```python
from build123d import *

# Parameters (mm, degrees)
F1_DEPTH = 35
F3_DEPTH = 70
F4_R     = 15
F5_DEPTH = 80.001
F7_DEPTH = 60.001


with BuildPart() as f1:
    # F0 (on Front) → F1 (new body, symmetric)
    with BuildSketch(Plane.XZ):
        Polygon((0, 20), (0, 0), (80, 0), (80, 80), (20, 80), (20, 20), align=None)
    extrude(amount=F1_DEPTH, both=True)

    # F2 (on face) → F3 (cut, through all)
    with BuildSketch(Plane.XZ.offset(35)):
        with BuildLine():
            Line((80, 40), (55, 40))
            ThreePointArc((55, 40), (40, 25), (55, 10))
            Line((55, 10), (80, 10))
            Line((80, 10), (80, 40))
        make_face()
    extrude(amount=-F3_DEPTH, mode=Mode.SUBTRACT)

    # F4 (on face) → F5 (cut, through all)
    with BuildSketch(Plane.XY.offset(80)):
        with Locations((20, 10)):
            Circle(F4_R)
    extrude(amount=-F5_DEPTH, mode=Mode.SUBTRACT)

    # F6 (on face) → F7 (cut, through all)
    with BuildSketch(Plane(origin=(20, 0, 0), x_dir=(0, -1, 0), z_dir=(-1, 0, 0))):
        Polygon((35, 80), (15, 80), (35, 50), align=None)
    extrude(amount=-F7_DEPTH, mode=Mode.SUBTRACT)


solid = f1.part
```
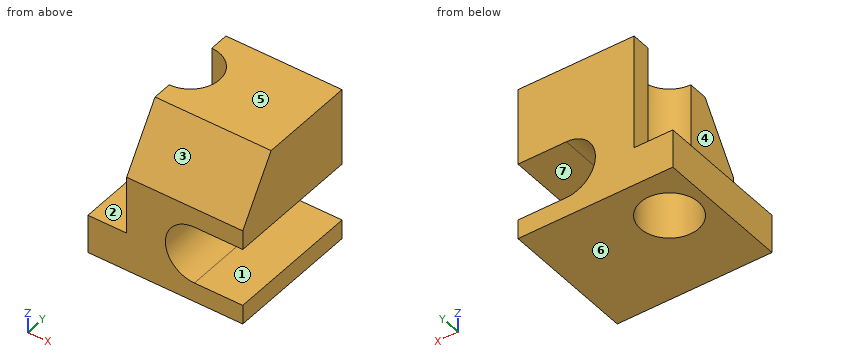
Model file for the job. Use its own axes, mm. Face numbers are marked on the shaded views. A direction names the side the tool comes from. Round coordinates to 2 decimals unless told otherwise and drop trailing zeros. Write each loop counter-clockwise with the first axis right and the second up, starting at its lowest first coordinate (ties: lowest second). Pieces come first, ordered by that corner, then holes. Notation, with made-up numbers: (68, 12) - (113, 12) arc R11 ccw to (113, 29) - close; hole circle Ø2 at (79.25, -27). An arc over 180 degrees is marked (long way). Use CSV: the item, a comma, the result in double quotes. Start each with the question number.
Item 1: Two-plate mould, pull along Z, no slides. Class the marked faces 4, 5, 6 and 7: released by +Z, released by -Z, zero draft, split by the parting line, or undercut.
Item 2: Band-saw the part on B-B (y = 10). Write the cut outline in (x, z).
Item 3: Pin check, flat tips, straight feed: P1, Ø24, axis at y = -23.5, z = 57.5, coming from the -X side; P2, Ø16, axis at x = 7, y = -14, coming from the +Z side. Stop position of each tip, or through.
Item 4: Band-saw the part on C-C (z = 25). Write the cut outline in (x, y), and give its area (3 significant figures).
Item 5: Tool access for the marked faces 1, 2 and 3: list every direction of +Z, -Z, +X, -X, +Y, -Y with a clear straight run to the whole face (end or side of a thin tool).
Item 6: Band-saw the part on A-A (x = 8). Write the cut outline in (y, z).
Item 7: Drill centre lines: L1, parallel to Z at x = 72, y = 22.5; L2, parallel to X at y = 10, z = 61; L3, parallel to X at y = -17, z = 46.5. Where is each one in solid material? Low to high. Write a range as [from, to].
Item 8: Band-saw the part on D-D (x = 60). Write the cut outline in (y, z).
Checked values:
1,face 4,"zero draft"
1,face 5,"released by +Z"
1,face 6,"released by -Z"
1,face 7,"undercut"
2,outline,"(0, 0) - (5, 0) - (5, 20) - (0, 20) - close; (35, 0) - (80, 0) - (80, 10) - (55, 10) arc R15 cw to (55, 40) - (80, 40) - (80, 80) - (35, 80) - close"
3,P1,"stops at x = 20"
3,P2,"stops at z = 20"
4,outline,"(20, -35) - (40, -35) - (40, 35) - (20, 35) - (20, 25) arc R15 cw to (20, -5) - close"
4,area,"1,050 mm²"
5,face 1,"+X, +Y, -Y"
5,face 2,"+Z, -X, +Y, -Y"
5,face 3,"+Z, +X, -X, -Y"
6,outline,"(-35, 0) - (1, 0) - (1, 20) - (-35, 20) - close; (19, 0) - (35, 0) - (35, 20) - (19, 20) - close"
7,L1,"z = [0, 10], [40, 80]"
7,L2,"x = [35, 80]"
7,L3,"x = [20, 80]"
8,outline,"(-35, 0) - (35, 0) - (35, 10) - (-35, 10) - close; (-35, 40) - (35, 40) - (35, 80) - (-15, 80) - (-35, 50) - close"
